```python
from build123d import *

# Parameters (mm, degrees)
EXTRUDE_START              = 0.3
EXTRUDE_1_DEPTH            = 4
EXTRUDE_2_DEPTH            = 4
SKETCH_3_W                 = 254.6
SKETCH_3_H                 = 12.878514778
EXTRUDE_3_DEPTH            = 3.4
CUT_EXTRUDE_1_REACH        = 253.212
SKETCH_4_W                 = 207.3
SKETCH_4_H                 = 7.3
SKETCH_5_W                 = 2.745808793
SKETCH_5_H                 = 3.85924733
SKETCH_5_H_2               = 3.447603815
EXTRUDE_4_DEPTH            = 2
SKETCH_6_W                 = 2.745808793
SKETCH_6_H                 = 3.85924733
SKETCH_6_H_2               = 3.447603815
EXTRUDE_5_DEPTH            = 2
CHAMFER_1_SIZE             = 3.464101615
CHAMFER_1_SIZE_2           = 2
CHAMFER_2_SIZE             = 2.7
CHAMFER_2_SIZE2            = 3.334222323
EXTRUDE_START_2            = -4
SKETCH_7_W                 = 20.333516096
SKETCH_7_H                 = 2
EXTRUDE_6_DEPTH            = 8
EXTRUDE_7_DEPTH            = 4
EXTRUDE_7_DEPTH_BACK       = 4
CUT_EXTRUDE_1_2_DEPTH      = 256.045082384
CUT_EXTRUDE_1_2_DEPTH_BACK = 1
SKETCH_9_W                 = 12.804262888
SKETCH_9_H                 = 1


with BuildPart() as part:
    # Sketch 1 → Extrude 1 (new body)
    with BuildSketch(Plane.XY.offset(EXTRUDE_START)):
        with BuildLine():
            Line((7.529253208, 6.254669476), (-12.804262888, 6.254669476))
            Line((-12.804262888, 6.254669476), (-12.804262888, -6.623845302))
            Line((-12.804262888, -6.623845302), (7.529253208, -6.623845302))
            Line((7.529253208, -6.623845302), (7.529253208, -2.63))
            Line((7.529253208, -2.63), (0, -2.63))
            ThreePointArc((0, -2.63), (-2.63, 0), (0, 2.63))
            Line((0, 2.63), (7.529253208, 2.63))
            Line((7.529253208, 2.63), (7.529253208, 6.254669476))
        make_face()
    extrude(amount=EXTRUDE_1_DEPTH)



with BuildPart() as body_2:
    # Sketch 2 → Extrude 2 (new body)
    with BuildSketch(Plane(origin=(0, 0, -246.3), x_dir=(-1, 0, 0), z_dir=(0, 0, -1))):
        with BuildLine():
            Line((-7.529253208, 6.254669476), (-7.529253208, 2.63))
            Line((-7.529253208, 2.63), (0, 2.63))
            ThreePointArc((0, 2.63), (2.63, 0), (0, -2.63))
            Line((0, -2.63), (-7.529253208, -2.63))
            Line((-7.529253208, -2.63), (-7.529253208, -6.623845302))
            Line((-7.529253208, -6.623845302), (12.804262888, -6.623845302))
            Line((12.804262888, -6.623845302), (12.804262888, 6.254669476))
            Line((12.804262888, 6.254669476), (-7.529253208, 6.254669476))
        make_face()
    extrude(amount=EXTRUDE_2_DEPTH)


with BuildPart() as part_1:
    add(part.part)

    add(body_2.part)  # Extrude 3 merges body 2
    # Sketch 3 → Extrude 3 (add)
    with BuildSketch(Plane.ZY.offset(12.804262888)):
        with Locations((-123, -0.184587913)):
            Rectangle(SKETCH_3_W, SKETCH_3_H)
    extrude(amount=-EXTRUDE_3_DEPTH)

    # Sketch 4 → Cut-Extrude 1 (cut, up to next)
    with BuildSketch(Plane.ZY.offset(12.804262888), mode=Mode.PRIVATE) as cut_extrude_1_sk1:
        with Locations((-120.8, -0.25)):
            Rectangle(SKETCH_4_W, SKETCH_4_H)
    cut_extrude_1_tool1 = extrude(cut_extrude_1_sk1.sketch, amount=-CUT_EXTRUDE_1_REACH, mode=Mode.PRIVATE) & part_1.part
    add(cut_extrude_1_tool1.solids().sort_by_distance((-12.804263, -0.25, -120.8))[0], mode=Mode.SUBTRACT)

    # Sketch 5 → Extrude 4 (add)
    with BuildSketch(Plane.XY.offset(-246.3)):
        with Locations((-1.372904397, -4.694221637)):
            Rectangle(SKETCH_5_W, SKETCH_5_H)
        with Locations((-1.372904397, 4.530867568)):
            Rectangle(SKETCH_5_W, SKETCH_5_H_2)
    extrude(amount=EXTRUDE_4_DEPTH)

    # Sketch 6 → Extrude 5 (add)
    with BuildSketch(Plane(origin=(0, 0, 0.3), x_dir=(-1, 0, 0), z_dir=(0, 0, -1))):
        with Locations((1.372904397, -4.694221637)):
            Rectangle(SKETCH_6_W, SKETCH_6_H)
        with Locations((1.372904397, 4.530867568)):
            Rectangle(SKETCH_6_W, SKETCH_6_H_2)
    extrude(amount=EXTRUDE_5_DEPTH)

    # Chamfer 1
    # the kernel refuses this chamfer: 3.464101615, 2 mm, written as the material it takes off along each edge
    with BuildSketch(Plane(origin=(-2.745808793, 15.216597417, -244.3), x_dir=(0.9998132206222079, 0, 0.01932676561270368), z_dir=(0, -1, 0))) as chamfer_1_piece_1_section:
        Polygon((CHAMFER_1_SIZE * 0.999813220662, -CHAMFER_1_SIZE * 0.0193267656135), (-CHAMFER_1_SIZE_2 * 0.0193267656127, -CHAMFER_1_SIZE_2 * 0.999813220622), (0, 0), align=None)
    chamfer_1_piece_1 = extrude(amount=21.371459697, mode=Mode.PRIVATE)
    chamfer_1_piece_1 = split(chamfer_1_piece_1, bisect_by=Plane(origin=(-1.581226814, 4.530867568, -246.3), z_dir=(0, 0, 1)), keep=Keep.TOP, mode=Mode.PRIVATE)
    add(chamfer_1_piece_1, mode=Mode.SUBTRACT)
    with BuildSketch(Plane(origin=(-2.745808793, -15.585773243, -244.3), x_dir=(-0.057893862402670956, 0, -0.9983227437537926), z_dir=(0, 1, 0))) as chamfer_1_piece_2_section:
        Polygon((CHAMFER_1_SIZE_2 * 0.998322743754, -CHAMFER_1_SIZE_2 * 0.0578938624027), (-CHAMFER_1_SIZE * 0.057893862405, -CHAMFER_1_SIZE * 0.998322743793), (0, 0), align=None)
    chamfer_1_piece_2 = extrude(amount=21.783103212, mode=Mode.PRIVATE)
    chamfer_1_piece_2 = split(chamfer_1_piece_2, bisect_by=Plane(origin=(-1.581226814, -4.694221637, -246.3), z_dir=(0, 0, 1)), keep=Keep.TOP, mode=Mode.PRIVATE)
    add(chamfer_1_piece_2, mode=Mode.SUBTRACT)
    with BuildSketch(Plane(origin=(-2.745808793, 6.197329969, -1.7), x_dir=(-0.057893862402671255, 0, 0.9983227437537926), z_dir=(0, -1, 0))) as chamfer_1_piece_3_section:
        Polygon((CHAMFER_1_SIZE_2 * 0.998322743754, -CHAMFER_1_SIZE_2 * 0.0578938624027), (-CHAMFER_1_SIZE * 0.057893862405, -CHAMFER_1_SIZE * 0.998322743793), (0, 0), align=None)
    chamfer_1_piece_3 = extrude(amount=21.783103212, mode=Mode.PRIVATE)
    chamfer_1_piece_3 = split(chamfer_1_piece_3, bisect_by=Plane(origin=(-1.581226814, -4.694221637, 0.3), z_dir=(0, 0, -1)), keep=Keep.TOP, mode=Mode.PRIVATE)
    add(chamfer_1_piece_3, mode=Mode.SUBTRACT)
    with BuildSketch(Plane(origin=(-2.745808793, 15.216597417, -1.7), x_dir=(-0.057893862402671255, 0, 0.9983227437537926), z_dir=(0, -1, 0))) as chamfer_1_piece_4_section:
        Polygon((CHAMFER_1_SIZE_2 * 0.998322743754, -CHAMFER_1_SIZE_2 * 0.0578938624027), (-CHAMFER_1_SIZE * 0.057893862405, -CHAMFER_1_SIZE * 0.998322743793), (0, 0), align=None)
    chamfer_1_piece_4 = extrude(amount=21.371459697, mode=Mode.PRIVATE)
    chamfer_1_piece_4 = split(chamfer_1_piece_4, bisect_by=Plane(origin=(-1.581226814, 4.530867568, 0.3), z_dir=(0, 0, -1)), keep=Keep.TOP, mode=Mode.PRIVATE)
    add(chamfer_1_piece_4, mode=Mode.SUBTRACT)

    # Chamfer 2
    chamfer_2_edges = [part_1.edges().sort_by_distance(p)[0] for p in [
        (-9.404262888, 6.254669476, -123),
        (-9.404262888, -6.623845302, -123),
    ]]
    chamfer_2_side = [part_1.faces().sort_by_distance(p)[0] for p in [
        (-9.404262888, -4.154484734, -123),
    ]]
    chamfer(chamfer_2_edges, length=CHAMFER_2_SIZE, length2=CHAMFER_2_SIZE2, reference=chamfer_2_side[0])

    # Sketch 7 → Extrude 6 (add)
    with BuildSketch(Plane.XY.offset(-246.3).offset(EXTRUDE_START_2)):
        with Locations((-2.63750484, -6.93)):
            Rectangle(SKETCH_7_W, SKETCH_7_H)
        with Locations((-2.63750484, 6.63)):
            Rectangle(SKETCH_7_W, SKETCH_7_H)
    extrude(amount=EXTRUDE_6_DEPTH)

    # Sketch 8 → Extrude 7 (add, two sides: drawn at the far end of the back side and taken through both)
    with BuildSketch(Plane(origin=(0, 0, 0.3), x_dir=(-1, 0, 0), z_dir=(0, 0, -1)).offset(-EXTRUDE_7_DEPTH_BACK)):
        Polygon((12.738485211, -6.623845302), (11.88165762, -5.93), (-7.529253208, -5.93), (-7.529253208, -7.93), (12.804262888, -7.93), (12.804262888, -6.623845302), align=None)
        Polygon((12.738485211, 6.254669476), (12.804262888, 6.254669476), (12.804262888, 7.63), (-7.529253208, 7.63), (-7.529253208, 5.63), (11.967082651, 5.63), align=None)
    extrude(amount=EXTRUDE_7_DEPTH + EXTRUDE_7_DEPTH_BACK)

    # Sketch 9 → Cut-Extrude 1 2 (cut, two sides: drawn at the far end of the back side and taken through both)
    with BuildSketch(Plane(origin=(0, 0, -250.3), x_dir=(-1, 0, 0), z_dir=(0, 0, -1)).offset(-CUT_EXTRUDE_1_2_DEPTH_BACK)):
        with Locations((6.402131444, 0)):
            Rectangle(SKETCH_9_W, SKETCH_9_H)
    extrude(amount=CUT_EXTRUDE_1_2_DEPTH + CUT_EXTRUDE_1_2_DEPTH_BACK, mode=Mode.SUBTRACT)


solid = part_1.part
```
Build history of the part. All positions in model axes, mm. A direction names the side the tool comes from. Round coordinates to 2 decimals unless told otherwise and drop trailing zeros. Write each loop counter-clockwise with the first axis right and the second up, starting at its lowest first coordinate (ties: lowest second). Pieces come first, ordered by that corner, then holes. Notation, with made-up numbers: (58, 89) - (80, 89) arc R29 cw to (80, 112) - close; hole circle Ø4 at (-18.5, -37). An arc over 180 degrees is marked (long way). Write each question's results on one line, items separated by ' | '. Start each with the question number.
Item 1: Saw through at C-C (x = -6.75). Write the cut outline in (y, z), and give its area (3 significant figures).
Item 2: Saw through at B-B (x = 2.25). Write the cut outline in (y, z), and give its area (3 significant figures).
Item 3: Drop flat-ended pins along their axis: P1, Ø0.8, axis at y = -5, z = -245.5, coming from the +X side; P2, Ø1, axis at x = -10.5, z = -79, coming from the +Y side; P3, Ø8, axis at y = 2, z = -177, coming from the +X side; P4, Ø6, axis at x = -4.5, z = -110, coming from the +Y side. Give the stop position or say it passes through.
Item 4: Wall check: L1, parallel to Z at x = 1, y = -4; L2, parallel to Z at x = -1.25, y = 5; L3, parallel to Y at x = -10.25, z = -164.5. Give the ranges that are in metal, low to high. Write a range as [from, to].
Item 5: Mould opens along X. For faces 4 (the face through (-2.63, 0.06, -248.27)), 5 (the face through (4, -2.63, 2)), 6 (the face through (-2, -5.93, -244)), 7 (the face through (-5, 0, 0.3)) say: pulls with the +X half, pulls with the -X half, needs draft (parallel to the pull), parting line crosses it, or undercut.
Item 6: Which spindle directions (+Z, -Z, +X, -X, +Y, -Y) get a long thin tool onto all of the face, cutting with end or side? Do faces 1 (the face through (-2, 5.63, -244)), 2 (the face through (4, 2.63, -248)), 3 (the face through (-3, -7.93, -246)). Say none if no direction does.
Results are:
1) outline: (-7.93, -250.3) - (-0.5, -250.3) - (-0.5, -249.3) - (0.5, -249.3) - (0.5, -250.3) - (7.63, -250.3) - (7.63, -242.3) - (5.63, -242.3) - (5.63, -246.3) - (-5.93, -246.3) - (-5.93, -242.3) - (-7.93, -242.3) - close; (-7.93, -3.7) - (-5.93, -3.7) - (-5.93, 0.3) - (5.63, 0.3) - (5.63, -3.7) - (7.63, -3.7) - (7.63, 4.3) - (-7.93, 4.3) - close | area: 155 mm²
2) outline: (-7.93, -250.3) - (-2.63, -250.3) - (-2.63, -246.3) - (-5.93, -246.3) - (-5.93, -242.3) - (-7.93, -242.3) - close; (-7.93, -3.7) - (-5.93, -3.7) - (-5.93, 0.3) - (-2.63, 0.3) - (-2.63, 4.3) - (-7.93, 4.3) - close; (2.63, -250.3) - (7.63, -250.3) - (7.63, -242.3) - (5.63, -242.3) - (5.63, -246.3) - (2.63, -246.3) - close; (2.63, 0.3) - (5.63, 0.3) - (5.63, -3.7) - (7.63, -3.7) - (7.63, 4.3) - (2.63, 4.3) - close | area: 114 mm²
3) P1: stops at x = 0 | P2: stops at y = 4.85 | P3: stops at x = -9.4 | P4: passes through
4) L1: z = [-250.3, -246.3], [0.3, 4.3] | L2: z = [-250.3, -245.44], [-0.56, 4.3] | L3: y = [-4.61, -3.9], [3.4, 4.24]
5) face 4: pulls with the +X half | face 5: needs draft | face 6: undercut | face 7: undercut
6) face 1: none | face 2: +Z, -Z, +X | face 3: +Z, -Z, +X, -X, -Y
